from build123d import *

# Parameters (mm, degrees)
F0_W     = 50
F0_H     = 777
F1_DEPTH = 12
F2_W     = 6
F2_H     = 777
F3_DEPTH = 6
F5_DEPTH = 12
F7_DEPTH = 12


with BuildPart() as f1:
    # F0 (on Top) → F1 (new body)
    with BuildSketch(Plane.XY):
        Rectangle(F0_W, F0_H)
    extrude(amount=F1_DEPTH)

    # F2 (on face) → F3 (cut)
    with BuildSketch(Plane(origin=(0, 0, 0), x_dir=(1, 0, 0), z_dir=(0, 0, -1))):
        with Locations((-22, 0)):
            Rectangle(F2_W, F2_H)
    extrude(amount=-F3_DEPTH, mode=Mode.SUBTRACT)

    # F4 (on face) → F5 (cut, through all)
    with BuildSketch(Plane.XY.offset(12)):
        Polygon((25, -338.5), (-25, -388.5), (25, -388.5), align=None)
    extrude(amount=-F5_DEPTH, mode=Mode.SUBTRACT)

    # F6 (on face) → F7 (cut, through all)
    with BuildSketch(Plane.XY.offset(12)):
        Polygon((25, 388.5), (-25, 388.5), (25, 338.5), align=None)
    extrude(amount=-F7_DEPTH, mode=Mode.SUBTRACT)


solid = f1.part
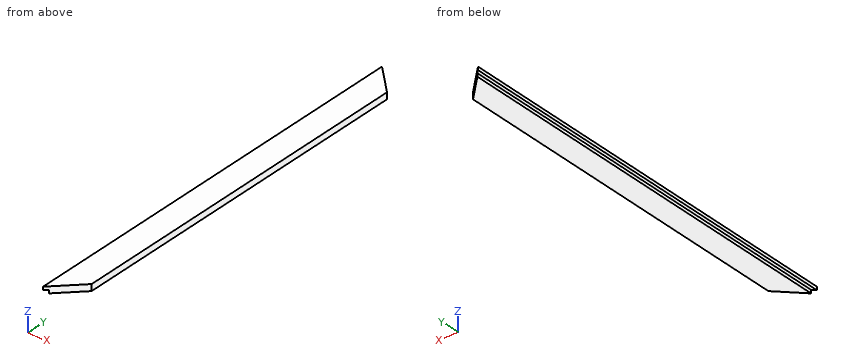
Geometry: final body of the model. Coordinates: model frame, mm. Give positions to 0.01 mm unless a question says otherwise; leave off trailing zeros. Write each loop counter-clockwise with the first axis right and the second up, starting at its lowest first coordinate (ties: lowest second). Pieces come first, ordered by that corner, then holes. Notation, with made-up numbers: M 38,-2 L 79,-2 A37 ccw 79,34 Z; hole C -38,14.25 d7. An arc over 180 degrees is marked long. Answer in a Markdown table with one row per item. Add a question column.
(1) First-contact query: pin 1 (6.5 mm diameter, centred on y = -85.5, z = 2.5, fed in from -X); pin 2 (6 mm diameter, centred on x = -6.5, z = 3.5, fed in from -Y); pin 3 (3 mm diameter, centred on x = -5, z = 1.5, fed in from -Y). Flat tips, straight axial feed; report the tip coordinate or a pass-through.
(2) Section A-A on y = 184. Return loops of the section in (x, z), and give its area (3 significant figures).
(3) Ray query, line 1 (X direction, y = 144, z = 4.25); line 2 (Z direction, x = -21, y = 144.5); line 3 (Y direction, x = 6.5, z = 3.5). Return the intervals inside material, ascending.
(4) Section B-B on x = 8.5. Return loops of the section in (y, z).
(5) Section C-C on z = 8. Return loops of the section in (x, y).
Result set:
| question | item | result |
|---|---|---|
| 1 | pin 1 | stops at x = -19 |
| 1 | pin 2 | stops at y = -373 |
| 1 | pin 3 | stops at y = -370 |
| 2 | outline | M -25,6 L -19,6 L -19,0 L 25,0 L 25,12 L -25,12 Z |
| 2 | area | 564 mm^2 |
| 3 | line 1 | x = -19 to 25 |
| 3 | line 2 | z = 6 to 12 |
| 3 | line 3 | y = -357 to 357 |
| 4 | outline | M -355,0 L 355,0 L 355,12 L -355,12 Z |
| 5 | outline | M -25,-388.5 L 25,-338.5 L 25,338.5 L -25,388.5 Z |
